```python
from build123d import *

# Parameters (mm, degrees)
SKETCH1_W               = 43.25
SKETCH1_H               = 48
SKETCH1_R               = 1.825
BOSS_EXTRUDE1_DEPTH     = 1.6
BOSS_EXTRUDE2_DEPTH     = 3
SKETCH3_W               = 24.55
SKETCH3_H               = 2.85
CUT_EXTRUDE1_DEPTH      = 21.6
SKETCH5_W               = 15
SKETCH5_H               = 2.65
BOSS_EXTRUDE4_DEPTH     = 2.4
SKETCH6_W               = 0.64
SKETCH6_H               = 0.64
BOSS_EXTRUDE5_DEPTH     = 5.7
FILLET1_R               = 2
CROQUIS1_W              = 1
CROQUIS1_H              = 1.5
CROQUIS1_W_2            = 10
CROQUIS1_H_2            = 4
CROQUIS1_W_3            = 1.267972753
CROQUIS1_H_3            = 0.734089488
CROQUIS1_H_4            = 0.798121905
CROQUIS1_W_4            = 1.14017415
CROQUIS1_H_5            = 2.245070142
CROQUIS1_W_5            = 1.862284445
CROQUIS1_H_6            = 2.017035312
CROQUIS1_W_6            = 0.931142223
CROQUIS1_H_7            = 0.646098685
CROQUIS1_W_7            = 0.570576299
CROQUIS1_H_8            = 0.403366405
SALIENTE_EXTRUIR1_DEPTH = 1.8


with BuildPart() as part:
    # Sketch1 → Boss-Extrude1 (new body)
    with BuildSketch(Plane(origin=(0, 0, 0), x_dir=(1, 0, 0), z_dir=(0, 1, 0))):
        with Locations((21.625, 24)):
            Rectangle(SKETCH1_W, SKETCH1_H)
        with Locations((3.8, 44.325)):
            Circle(SKETCH1_R, mode=Mode.SUBTRACT)
        with Locations((3.8, 3.675)):
            Circle(SKETCH1_R, mode=Mode.SUBTRACT)
        with Locations((39.45, 44.325)):
            Circle(SKETCH1_R, mode=Mode.SUBTRACT)
        with Locations((39.45, 3.675)):
            Circle(SKETCH1_R, mode=Mode.SUBTRACT)
    extrude(amount=BOSS_EXTRUDE1_DEPTH)

    # Sketch2 → Boss-Extrude2 (add)
    with BuildSketch(Plane(origin=(0, 1.6, 0), x_dir=(1, 0, 0), z_dir=(0, 1, 0))):
        with BuildLine():
            Line((6.75, 0), (11.8, 0))
            ThreePointArc((11.8, 0), (21.175, 6.86), (30.55, 0))
            Line((30.55, 0), (35.6, 0))
            Line((35.6, 0), (35.6, 29.5))
            Line((35.6, 29.5), (6.75, 29.5))
            Line((6.75, 29.5), (6.75, 0))
        make_face()
    extrude(amount=BOSS_EXTRUDE2_DEPTH)

    # Sketch3 → Cut-Extrude1 (cut)
    with BuildSketch(Plane.XY):
        with Locations((20.525, 3.025)):
            Rectangle(SKETCH3_W, SKETCH3_H)
    extrude(amount=-CUT_EXTRUDE1_DEPTH, mode=Mode.SUBTRACT)

    # Sketch5 → Boss-Extrude4 (add)
    with BuildSketch(Plane(origin=(0, 1.6, 0), x_dir=(1, 0, 0), z_dir=(0, 1, 0))):
        with Locations((24.293988912, 44.375)):
            Rectangle(SKETCH5_W, SKETCH5_H)
    extrude(amount=BOSS_EXTRUDE4_DEPTH)

    # Sketch6 → Boss-Extrude5 (add)
    with BuildSketch(Plane(origin=(0, 4, 0), x_dir=(1, 0, 0), z_dir=(0, 1, 0))):
        with Locations((18.153988912, 44.34)):
            Rectangle(SKETCH6_W, SKETCH6_H)
        with Locations((20.653988912, 44.34)):
            Rectangle(SKETCH6_W, SKETCH6_H)
        with Locations((23.153988912, 44.34)):
            Rectangle(SKETCH6_W, SKETCH6_H)
        with Locations((25.653988912, 44.34)):
            Rectangle(SKETCH6_W, SKETCH6_H)
        with Locations((28.153988912, 44.34)):
            Rectangle(SKETCH6_W, SKETCH6_H)
        with Locations((30.653988912, 44.34)):
            Rectangle(SKETCH6_W, SKETCH6_H)
    extrude(amount=BOSS_EXTRUDE5_DEPTH)

    # Fillet1
    fillet1_edges = [part.edges().sort_by_distance(p)[0] for p in [
        (0, 0.8, 0),
        (43.25, 0.8, 0),
        (43.25, 0.8, -48),
        (0, 0.8, -48),
    ]]
    fillet(fillet1_edges, radius=FILLET1_R)

    # Croquis1 → Saliente-Extruir1 (add)
    with BuildSketch(Plane(origin=(0, 1.6, 0), x_dir=(1, 0, 0), z_dir=(0, 1, 0))):
        with Locations((37.688468842, 26.759910401)):
            Rectangle(CROQUIS1_W, CROQUIS1_H)
        with Locations((19.480186858, 38.116576041)):
            Rectangle(CROQUIS1_W_2, CROQUIS1_H_2)
        with Locations((30.396581675, 39.749531297)):
            Rectangle(CROQUIS1_W_3, CROQUIS1_H_3)
        with Locations((30.396581675, 38.498601682)):
            Rectangle(CROQUIS1_W_3, CROQUIS1_H_4)
        with Locations((33.151840343, 38.99404097)):
            Rectangle(CROQUIS1_W_4, CROQUIS1_H_5)
        with Locations((37.237464381, 39.108058385)):
            Rectangle(CROQUIS1_W_5, CROQUIS1_H_6)
        with Locations((36.771893269, 37.244410117)):
            Rectangle(CROQUIS1_W_6, CROQUIS1_H_7)
        with Locations((32.867041418, 36.787844886)):
            Rectangle(CROQUIS1_W_7, CROQUIS1_H_8)
        with Locations((37.688468842, 28.759910401)):
            Rectangle(CROQUIS1_W, CROQUIS1_H)
        with Locations((31.277047992, 36.787844886)):
            Rectangle(CROQUIS1_W_7, CROQUIS1_H_8)
    extrude(amount=SALIENTE_EXTRUIR1_DEPTH)


solid = part.part
```
Design review of the part built by this model. Coordinates are the model's own, in mm. A direction names the side the tool comes from. Give positions to 0.01 mm unless a question says otherwise; leave off trailing zeros. Order: outer loops, then holes, each group sorted by start corner. A loop starts at its lowest first (then second) coordinate and runs counter-clockwise, first axis right, second up. Notation, with made-up numbers: (-21.5, 8.5) -> (21.5, 8.5) arc R15 ccw to (21.5, 29.5) -> close; hole circle Ø5 at (-32, 36.5). An arc over 180 degrees is marked (long way). Write each question's results on one line, items separated by ' | '. Start each with the question number.
Q1. Machinability: for faces 4 (the flat face through (20, 1.6, -11)), 5 (the flat face through (6.75, 3, -15)), 6 (the flat face through (33.722, 2, -39)), 7 (the flat face through (24, 3, -45.7)), which of the approach directions +Z, -Z, +X, -X, +Y, -Y give a long, thin tool a straight path to every point of the face, cutting with its end or side? Answer none if there is none.
Q2. For pin 1 (0.9 mm diameter, centred on y = 2.5, z = -38, fed in from +X); pin 2 (0.9 mm diameter, centred on y = 3, z = -7.5, fed in from +X); pin 3 (8 mm diameter, centred on x = 8.5, z = -41.5, fed in from +Y); pin 4 (10 mm diameter, centred on x = 24.5, z = -37, fed in from -Y), all flat-tipped, find the tip position at first contact; note any pin that passes through.
Q3. Add section C-C on z = -10.5. Give the boundary of the cut face in (x, y), and give its area (3 significant figures).
Q4. Mouldability with a two-part tool opening along Y and no side actions: class faces 1 (the cylindrical face through (0.57, 0.81, -0.6)), 2 (the flat face through (20, 3, -21.6)), 3 (the flat face through (19, 3.4, -38)) as +Y half, -Y half, draft (parallel to the pull), parting line (faces both ways), or undercut.
Q5. Wall thickness on L1, parallel to Z at x = 39.45, y = 0.9; L2, parallel to Z at x = 33.5, y = 1.75; L3, parallel to Z at x = 19.5, y = 3.5: over which ranges is each line inside the solid? List them lowest first. Write a range as from..to.
Q6. Add section A-A on y = 5.25. Give the boundary of the cut face in (x, z).
Q7. Add section B-B on x = 3.8. Give the boundary of the cut face in (y, z).
Q8. Add section D-D on y = 1. Give the boundary of the cut face in (x, z) (3 decimals), and give its area (3 significant figures).
Found:
1) face 4: +Z | face 5: +Z, -Z, -X, +Y | face 6: -Z, +Y | face 7: -Z, +X, -X, +Y
2) pin 1: stops at x = 38.17 | pin 2: stops at x = 35.6 | pin 3: stops at y = 1.6 | pin 4: stops at y = 0
3) outline: (0, 0) -> (43.25, 0) -> (43.25, 1.6) -> (35.6, 1.6) -> (35.6, 4.6) -> (6.75, 4.6) -> (6.75, 1.6) -> (0, 1.6) -> close; hole (8.25, 1.6) -> (32.8, 1.6) -> (32.8, 4.45) -> (8.25, 4.45) -> close | area: 85.8 mm2
4) face 1: draft | face 2: undercut | face 3: +Y half
5) L1: z = -48..-46.15, -42.5..-5.5, -1.85..0 | L2: z = -40.12..-37.87, -29.5..0 | L3: z = -45.7..-43.05, -29.5..-21.6
6) outline: (17.83, -44.66) -> (18.47, -44.66) -> (18.47, -44.02) -> (17.83, -44.02) -> close; (20.33, -44.66) -> (20.97, -44.66) -> (20.97, -44.02) -> (20.33, -44.02) -> close; (22.83, -44.66) -> (23.47, -44.66) -> (23.47, -44.02) -> (22.83, -44.02) -> close; (25.33, -44.66) -> (25.97, -44.66) -> (25.97, -44.02) -> (25.33, -44.02) -> close; (27.83, -44.66) -> (28.47, -44.66) -> (28.47, -44.02) -> (27.83, -44.02) -> close; (30.33, -44.66) -> (30.97, -44.66) -> (30.97, -44.02) -> (30.33, -44.02) -> close
7) outline: (0, -48) -> (1.6, -48) -> (1.6, -46.15) -> (0, -46.15) -> close; (0, -42.5) -> (1.6, -42.5) -> (1.6, -5.5) -> (0, -5.5) -> close; (0, -1.85) -> (1.6, -1.85) -> (1.6, 0) -> (0, 0) -> close
8) outline: (0, -46) arc R2 ccw to (2, -48) -> (41.25, -48) arc R2 ccw to (43.25, -46) -> (43.25, -2) arc R2 ccw to (41.25, 0) -> (2, 0) arc R2 ccw to (0, -2) -> close; hole circle Ø3.65 at (3.8, -44.325); hole circle Ø3.65 at (3.8, -3.675); hole circle Ø3.65 at (39.45, -44.325); hole circle Ø3.65 at (39.45, -3.675) | area: 2,030 mm2
